```python
from build123d import *

# Parameters (mm, degrees)
BOSS_EXTRUDE1_DEPTH = 12
CUT_EXTRUDE2_REACH  = 122
SKETCH3_R           = 2.5
CHAMFER2_SIZE       = 2.5


with BuildPart() as part:
    # Sketch1 → Boss-Extrude1 (new body)
    with BuildSketch(Plane.XY):
        with BuildLine():
            Line((120, 35), (120, 5))
            Line((120, 5), (120, -25))
            Line((120, -25), (113, -25))
            Line((113, -25), (113, -5))
            ThreePointArc((113, -5), (111.535533906, -1.464466094), (108, 0))
            Line((108, 0), (0, 0))
            Line((0, 0), (0, 20))
            ThreePointArc((0, 20), (7.5, 27.5), (15, 20))
            Line((15, 20), (12.5, 20))
            ThreePointArc((12.5, 20), (7.5, 25), (2.5, 20))
            Line((2.5, 20), (2.5, 10))
            Line((2.5, 10), (108, 10))
            ThreePointArc((108, 10), (111.535533906, 11.464466094), (113, 15))
            Line((113, 15), (113, 35))
            Line((113, 35), (120, 35))
        make_face()
    extrude(amount=BOSS_EXTRUDE1_DEPTH)

    # Sketch3 → Cut-Extrude2 (cut, up to next)
    with BuildSketch(Plane(origin=(120, 0, 0), x_dir=(0, 0, -1), z_dir=(1, 0, 0)), mode=Mode.PRIVATE) as cut_extrude2_sk1:
        with Locations((-6, 29)):
            Circle(SKETCH3_R)
    cut_extrude2_tool1 = extrude(cut_extrude2_sk1.sketch, amount=-CUT_EXTRUDE2_REACH, mode=Mode.PRIVATE) & part.part
    add(cut_extrude2_tool1.solids().sort_by_distance((120, 29, 6))[0], mode=Mode.SUBTRACT)
    # Sketch3 → Cut-Extrude2 (cut, up to next)
    with BuildSketch(Plane(origin=(120, 0, 0), x_dir=(0, 0, -1), z_dir=(1, 0, 0)), mode=Mode.PRIVATE) as cut_extrude2_sk2:
        with Locations((-6, -19)):
            Circle(SKETCH3_R)
    cut_extrude2_tool2 = extrude(cut_extrude2_sk2.sketch, amount=-CUT_EXTRUDE2_REACH, mode=Mode.PRIVATE) & part.part
    add(cut_extrude2_tool2.solids().sort_by_distance((120, -19, 6))[0], mode=Mode.SUBTRACT)

    # Chamfer2
    chamfer2_edges = [part.edges().sort_by_distance(p)[0] for p in [
        (113, 29, 8.5),
        (113, -19, 8.5),
    ]]
    chamfer(chamfer2_edges, length=CHAMFER2_SIZE)


solid = part.part
```
Part model, mm, in its own coordinate system. A direction names the side the tool comes from. Give positions to 0.01 mm unless a question says otherwise; leave off trailing zeros. Order: outer loops, then holes, each group sorted by start corner. A loop starts at its lowest first (then second) coordinate and runs counter-clockwise, first axis right, second up. Notation, with made-up numbers: M 37,-12.75 L 46,-12.75 A26 ccw 46,16.25 Z; hole C -28,19.5 d3. An arc over 180 degrees is marked long. Use a Markdown table: item, result. Add a question column.
(1) Probe line 1 along Y through (x, z) = (119, 6); line 2 along X through (y, z) = (19.5, 0.5); line 3 along Y through (x, z) = (79.5, 3). List the from-to ranges inside material, lowest first. Write a range as [from, to].
(2) Drop flat-ended pins along their axis: P1, Ø5, axis at y = 3.5, z = 7, coming from the -X side; P2, Ø6, axis at x = 54, z = 4.5, coming from the -Y side; P3, Ø6, axis at y = -16, z = 7, coming from the -X side; P4, Ø4.5, axis at y = 29, z = 6, coming from the +X side. Give the stop position or say it passes through.
(3) Saw through at B-B, the plane y = -19. Give the cut face in (x, z), and give its area (4 significant figures).
(4) Saw through at D-D, the plane x = 54. Give the cut face in (y, z).
(5) 3-axis set-ups, long thin cutter, end or side, ignore diameter. For faces 1 (the face through (55, 0, 6)), 2 (the face through (2.5, 15, 6)), 3 (the face through (115.34, 26.64, 4.77)), 4 (the face through (117.78, 31.11, 4.66)), 5 (the face through (111, 11, 6)): which of +Z, -Z, +X, -X, +Y, -Y reach the whole face in a straight line?
(6) Saw through at C-C, the plane x = 7.5. Give the cut face in (y, z).
(7) Mould opens along Y. For faces 6 (the face through (7.6, 25, 5.9)), 7 (the face through (112, -2, 6)), 8 (the face through (120, 5, 6)) say: +Y half, -Y half, draft (parallel to the pull), parting line (faces both ways), or undercut.
(8) Saw through at A-A, the plane z = 6. Give the cut face in (x, y), and give its area (3 significant figures).
Answer key:
| question | item | result |
|---|---|---|
| 1 | line 1 | [-25, -21.5], [-16.5, 26.5], [31.5, 35] |
| 1 | line 2 | [0, 2.5], [113, 120] |
| 1 | line 3 | [0, 10] |
| 2 | P1 | x = 0 |
| 2 | P2 | y = 0 |
| 2 | P3 | x = 113 |
| 2 | P4 | x = 10.77 |
| 3 | outline | M 113,0 L 120,0 L 120,3.5 L 115.5,3.5 L 113,1 Z; M 113,11 L 115.5,8.5 L 120,8.5 L 120,12 L 113,12 Z |
| 3 | area | 42.75 mm^2 |
| 4 | outline | M 0,0 L 10,0 L 10,12 L 0,12 Z |
| 5 | face 1 | +Z, -Z, -X, -Y |
| 5 | face 2 | +Z, -Z |
| 5 | face 3 | none |
| 5 | face 4 | +X |
| 5 | face 5 | +Z, -Z, +Y |
| 6 | outline | M 0,0 L 10,0 L 10,12 L 0,12 Z; M 25,0 L 27.5,0 L 27.5,12 L 25,12 Z |
| 7 | face 6 | undercut |
| 7 | face 7 | -Y half |
| 7 | face 8 | draft |
| 8 | outline | M 0,0 L 108,0 A5 cw 113,-5 L 113,-14 L 115.5,-16.5 L 120,-16.5 L 120,26.5 L 115.5,26.5 L 113,24 L 113,15 A5 cw 108,10 L 2.5,10 L 2.5,20 A5 cw 12.5,20 L 15,20 A7.5 ccw 0,20 Z; M 113,-25 L 120,-25 L 120,-21.5 L 115.5,-21.5 L 113,-24 Z; M 113,34 L 115.5,31.5 L 120,31.5 L 120,35 L 113,35 Z |
| 8 | area | 1,550 mm^2 |
